Geometry: final body of the model. Coordinates: model frame, mm. Face numbers are marked on the shaded views. A direction names the side the tool comes from. Give positions to 0.01 mm unless a question says otherwise; leave off trailing zeros. Loops run counter-clockwise (first coordinate to the right, second up) from the corner with the lowest first, then second, coordinate; pieces in that order, holes last. Notation, with made-up numbers: (-7.5, 44) - (35.5, 44) arc R11 cw to (35.5, 51) - close; hole circle Ø2 at (-15, 23.5). An arc over 180 degrees is marked (long way). Answer in a Markdown table with one row per item.
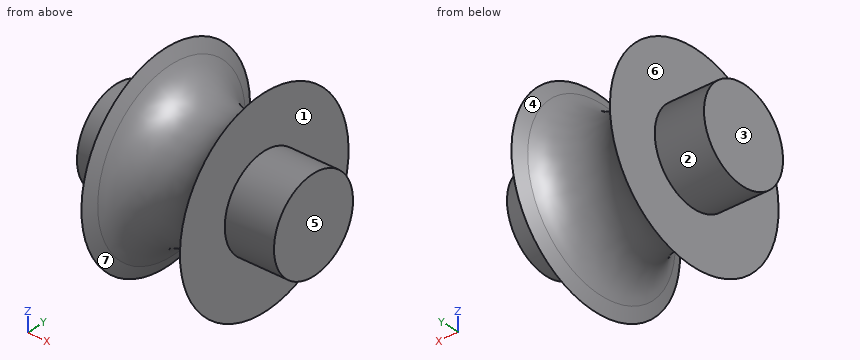
from build123d import *


with BuildPart() as f1:
    # F0 (on Front) → F1 (revolve)
    with BuildSketch(Plane.XZ):
        with BuildLine():
            Line((-25.4, 11.90625), (-25.4, 0))
            Line((-25.4, 0), (0, 0))
            Line((0, 0), (25.4, 0))
            Line((25.4, 0), (25.4, 11.90625))
            Line((25.4, 11.90625), (12.7, 11.90625))
            Line((12.7, 11.90625), (12.7, 25.4))
            Line((12.7, 25.4), (11.219473, 22.225))
            ThreePointArc((11.219473, 22.225), (0, 15.077407), (-11.219473, 22.225))
            Line((-11.219473, 22.225), (-12.7, 25.4))
            Line((-12.7, 25.4), (-12.7, 11.90625))
            Line((-12.7, 11.90625), (-25.4, 11.90625))
        make_face()
    revolve(axis=Axis((-5.579621, 0, 0), (1, 0, 0)))


solid = f1.part
Q1. First-contact query: pin 1 (4 mm diameter, centred on x = -14.5, z = 19.5, fed in from +Y); pin 2 (8 mm diameter, centred on y = 12, z = -6.5, fed in from +X); pin 3 (1.5 mm diameter, centred on y = -5.5, z = -16, fed in from +X); pin 4 (4 mm diameter, centred on y = -13.5, z = -11.5, fed in from -X). Flat tips, straight axial feed; report the tip coordinate or a pass-through.
Check values:
| item | result |
|---|---|
| pin 1 | y = 17.27 |
| pin 2 | x = 25.4 |
| pin 3 | x = 12.7 |
| pin 4 | x = -12.7 |
Q2. Draft query along X for the marked faces 5, 6 and 7. Return one class per face: pulls with the +X half, pulls with the -X half, needs draft (parallel to the pull), parting line crosses it, or undercut.
Check values:
| item | result |
|---|---|
| face 5 | pulls with the +X half |
| face 6 | pulls with the -X half |
| face 7 | undercut |
Q3. Material intervals for line 1 along X through (y, z) = (20.5, 8.5); line 2 along X through (y, z) = (-13, 20.5); line 3 along X through (y, z) = (-3, -14), sorted ascending.
Check values:
| item | result |
|---|---|
| line 1 | -12.7 to -11.2, 11.2 to 12.7 |
| line 2 | -12.7 to -12.18, 12.18 to 12.7 |
| line 3 | -12.7 to 12.7 |
Q4. Cut plane D-D (x = 10). Output: boundary loops of the cut face in (y, z).
Check values:
| item | result |
|---|---|
| outline | circle Ø40.32 at (0, 0) |
Q5. Cut plane C-C (x = 18.5). Output: boundary loops of the cut face in (y, z), and give its area (3 significant figures).
Check values:
| item | result |
|---|---|
| outline | circle Ø23.81 at (0, 0) |
| area | 445 mm² |
Q6. Reachability of the marked faces 1, 2, 3 and 4 from +Z, -Z, +X, -X, +Y, -Y: full face, straight path, thin tool, end or side. Return the list, or none.
Check values:
| item | result |
|---|---|
| face 1 | +X |
| face 2 | -X |
| face 3 | +Z, -Z, -X, +Y, -Y |
| face 4 | none |
Q7. Cut plane A-A (y = 0). Output: boundary loops of the cut face in (x, z) (3 decimals).
Check values:
| item | result |
|---|---|
| outline | (-25.4, -11.906) - (-12.7, -11.906) - (-12.7, -25.4) - (-11.219, -22.225) arc R12.379 cw to (11.219, -22.225) - (12.7, -25.4) - (12.7, -11.906) - (25.4, -11.906) - (25.4, 11.906) - (12.7, 11.906) - (12.7, 25.4) - (11.219, 22.225) arc R12.379 cw to (-11.219, 22.225) - (-12.7, 25.4) - (-12.7, 11.906) - (-25.4, 11.906) - close |
